Source: CAD feature listing. Evaluate the final solid. Frame: model axes, mm. A direction names the side the tool comes from. Round coordinates to 2 decimals unless told otherwise and drop trailing zeros. One line per item, written item: value.
from build123d import *

# Parameters (mm, degrees)
ZAOKR_GLENIE1_R  = 2
SFAZOWANIE1_SIZE = 0.5


with BuildPart() as part:
    # Szkic1 → Obrót1 (revolve)
    with BuildSketch(Plane(origin=(0, 0, 0), x_dir=(0, 0, -1), z_dir=(1, 0, 0)), mode=Mode.PRIVATE) as obr_t1_sk:
        Polygon((-5, 4), (5, 4), (5, 25), (4, 25), (1.5, 22), (-1.5, 22), (-4, 25), (-5, 25), align=None)
    revolve(obr_t1_sk.sketch.rotate(Axis((0, 0, 0), (0, 0, -1)), 90), axis=Axis((0, 0, 0), (0, 0, -1)))

    # Zaokrąglenie1
    zaokr_glenie1_edges = [part.edges().sort_by_distance(p)[0] for p in [
        (-22, 0, -1.5),
        (-22, 0, 1.5),
    ]]
    fillet(zaokr_glenie1_edges, radius=ZAOKR_GLENIE1_R)

    # Sfazowanie1
    sfazowanie1_edges = [part.edges().sort_by_distance(p)[0] for p in [
        (-4, 0, 5),
        (-4, 0, -5),
    ]]
    chamfer(sfazowanie1_edges, length=SFAZOWANIE1_SIZE)


solid = part.part
1. Reachability of faces 4 (the face through (0, 5, -5)), 5 (the face through (10.15, 19.52, 0.01)) from +Z, -Z, +X, -X, +Y, -Y: full face, straight path, thin tool, end or side. Return the list, or none.
Report:
face 4: -Z, +X, -X, +Y, -Y
face 5: none
2. Pull-direction query (Y, two-part tool) for faces 1 (the face through (23.846, -7.509, -4.493)), 2 (the face through (-0.867, 3.905, -0.063)), 3 (the face through (0, 5, 5)); classes: released by +Y, released by -Y, zero draft, split by the parting line, or undercut.
Report:
face 1: split by the parting line
face 2: undercut
face 3: zero draft
3. Pin query (flat end, axial travel): pin 1 (3 mm diameter, centred on y = -5.5, z = -0.5, fed in from -X); pin 2 (1 mm diameter, centred on y = 7.5, z = 2.5, fed in from -X); pin 3 (3 mm diameter, centred on y = -1, z = 1.5, fed in from +X). Return the tip coordinate at first contact, or that it passes through.
Report:
pin 1: stops at x = -21.97
pin 2: stops at x = -22.61
pin 3: stops at x = 23.78
4. Ray query, line 1 (Y direction, x = 0, z = 0.75); line 2 (Y direction, x = -3.5, z = 2); line 3 (Z direction, x = 20.5, y = 10.5). Return the intervals inside material, ascending. Write a range as [from, to].
Report:
line 1: y = [-22.01, -4], [4, 22.01]
line 2: y = [-22.34, -1.94], [1.94, 22.34]
line 3: z = [-5, -2.36], [2.36, 5]
